Can you work these out from the model? Positions are in its coordinate system, mm. A direction names the side the tool comes from. Give positions to 0.01 mm unless a question says otherwise; leave off trailing zeros. Loops run counter-clockwise (first coordinate to the right, second up) from the corner with the lowest first, then second, coordinate; pieces in that order, holes last. Notation, with made-up numbers: M 7.25,-32.75 L 32.25,-32.75 A23 ccw 32.25,-7.75 Z; hole C 5,51 d6. An arc over 180 degrees is marked long. Put each result on its own line as item: value. Start each with the question number.
1) Imagine slicing it at B-B (z = 899). Write out the boundary of the cut face in (x, y), then the cut area to 3 significant figures.
2) For faces 5 (the cylindrical face through (378.69, -92.32, 749.78)), 6 (the flat face through (-317, -41, 865)), 7 (the flat face through (1, -39, 965)), 8 (the flat face through (-1, -55, 426)), 9 (the flat face through (313, -41, 865)), which set-ups out of +Z, -Z, +X, -X, +Y, -Y let a thin tool reach every point of the face, with its end or its side?
3) Imagine slicing it at A-A (y = -152.5). Write out the boundary of the cut face in (x, z).
4) For P1, Ø23.5, axis at x = -300, z = 662.5, coming from the -Y side; P2, Ø1, axis at x = -307.5, z = 209, coming from the -Y side; P3, Ø3, axis at x = 303.5, y = -105.5, coming from the +Z side, each with a flat end and sliding along its axis, tell me the tip position at first contact or that it passes through.
5) Imagine slicing it at C-C (z = 471.5). Write out the boundary of the cut face in (x, y), then the cut area to 3 significant figures.
6) If we mould it in two halves opening along X, with no side actions, what happens to faces 1 (the flat face through (310.4, -110, 147.9)), 2 (the cylindrical face through (-12.042, -92.325, 941.713)), 3 (the flat face through (-465, -39, 456)), 4 (the cylindrical face through (293.491, -107.465, 774.575))? For each: +X half, -X half, draft (parallel to the pull), parting line (faces both ways), or undercut.
7) Please list where these lines run through material, in increasing order: line 1 along Z through (x, y) = (0, -92.75); line 2 along X through (y, z) = (-84, 662); line 3 along Z through (x, y) = (-300, -50.5). Write a range as from..to.
8) Imagine slicing it at D-D (z = 276). Write out the boundary of the cut face in (x, y).
from build123d import *

# Parameters (mm, degrees)
F0_W      = 690
F0_H      = 350
F0_H_2    = 200
F1_DEPTH  = 80
F2_R      = 25
F2_R_2    = 75
F3_DEPTH  = 100
F4_R      = 75
F5_DEPTH  = 150
F6_R      = 82.5
F6_R_2    = 9
F6_R_3    = 25
F7_DEPTH  = 25
F8_R      = 50
F8_R_2    = 25
F9_DEPTH  = 5
F10_R     = 75
F11_DEPTH = 25
F12_R     = 37.5
F13_DEPTH = 100
F14_R     = 92.5
F14_R_2   = 9
F14_R_3   = 37.5
F15_DEPTH = 25
F16_R     = 60
F16_R_2   = 37.5
F17_DEPTH = 5
F18_W     = 930
F18_H     = 1000
F19_DEPTH = 100
F20_R     = 7
F21_DEPTH = 50
F22_W     = 300
F22_H     = 100
F23_DEPTH = 80


with BuildPart() as f1:
    # F0 (on Front) → F1 (new body)
    with BuildSketch(Plane.XZ):
        Polygon((345, -965), (465, -965), (465, 965), (-465, 965), (-465, -965), (-345, -965), (-345, -765), (345, -765), align=None)
        with Locations((0, -470)):
            Rectangle(F0_W, F0_H, mode=Mode.SUBTRACT)
        with Locations((0, -75)):
            Rectangle(F0_W, F0_H_2, mode=Mode.SUBTRACT)
    extrude(amount=F1_DEPTH)

    # F2 (on face) → F3 (cut)
    with BuildSketch(Plane.XZ.offset(80)):
        with Locations((-300, 125)):
            Circle(F2_R)
        with Locations((0, 425)):
            Circle(F2_R_2)
        with Locations((-300, 725)):
            Circle(F2_R)
        with Locations((300, 125)):
            Circle(F2_R)
        with Locations((300, 725)):
            Circle(F2_R)
    extrude(amount=-F3_DEPTH, mode=Mode.SUBTRACT)

    # F4 (on face) → F5 (join)
    with BuildSketch(Plane.XZ.offset(80)):
        with Locations((-370, 415)):
            Circle(F4_R)
        with Locations((370, 415)):
            Circle(F4_R)
    extrude(amount=F5_DEPTH)

    # F6 (on face) → F7 (join)
    with BuildSketch(Plane.XZ.offset(80)):
        with Locations((-300, 725)):
            Circle(F6_R)
        with Locations((-300, 662.5)):
            Circle(F6_R_2, mode=Mode.SUBTRACT)
        with Locations((-362.5, 725)):
            Circle(F6_R_2, mode=Mode.SUBTRACT)
        with Locations((-300, 725)):
            Circle(F6_R_3, mode=Mode.SUBTRACT)
        with Locations((-300, 787.5)):
            Circle(F6_R_2, mode=Mode.SUBTRACT)
        with Locations((-237.5, 725)):
            Circle(F6_R_2, mode=Mode.SUBTRACT)
        with Locations((-300, 125)):
            Circle(F6_R)
        with Locations((-300, 62.5)):
            Circle(F6_R_2, mode=Mode.SUBTRACT)
        with Locations((-362.5, 125)):
            Circle(F6_R_2, mode=Mode.SUBTRACT)
        with Locations((-300, 125)):
            Circle(F6_R_3, mode=Mode.SUBTRACT)
        with Locations((-237.5, 125)):
            Circle(F6_R_2, mode=Mode.SUBTRACT)
        with Locations((-300, 187.5)):
            Circle(F6_R_2, mode=Mode.SUBTRACT)
        with Locations((300, 725)):
            Circle(F6_R)
        with Locations((300, 662.5)):
            Circle(F6_R_2, mode=Mode.SUBTRACT)
        with Locations((237.5, 725)):
            Circle(F6_R_2, mode=Mode.SUBTRACT)
        with Locations((300, 725)):
            Circle(F6_R_3, mode=Mode.SUBTRACT)
        with Locations((362.5, 725)):
            Circle(F6_R_2, mode=Mode.SUBTRACT)
        with Locations((300, 787.5)):
            Circle(F6_R_2, mode=Mode.SUBTRACT)
        with Locations((300, 125)):
            Circle(F6_R)
        with Locations((237.5, 125)):
            Circle(F6_R_2, mode=Mode.SUBTRACT)
        with Locations((300, 62.5)):
            Circle(F6_R_2, mode=Mode.SUBTRACT)
        with Locations((300, 125)):
            Circle(F6_R_3, mode=Mode.SUBTRACT)
        with Locations((362.5, 125)):
            Circle(F6_R_2, mode=Mode.SUBTRACT)
        with Locations((300, 187.5)):
            Circle(F6_R_2, mode=Mode.SUBTRACT)
    extrude(amount=F7_DEPTH)

    # F8 (on face) → F9 (join)
    with BuildSketch(Plane.XZ.offset(105)):
        with Locations((-300, 725)):
            Circle(F8_R)
        with Locations((-300, 725)):
            Circle(F8_R_2, mode=Mode.SUBTRACT)
        with Locations((-300, 125)):
            Circle(F8_R)
        with Locations((-300, 125)):
            Circle(F8_R_2, mode=Mode.SUBTRACT)
        with Locations((300, 725)):
            Circle(F8_R)
        with Locations((300, 725)):
            Circle(F8_R_2, mode=Mode.SUBTRACT)
        with Locations((300, 125)):
            Circle(F8_R)
        with Locations((300, 125)):
            Circle(F8_R_2, mode=Mode.SUBTRACT)
    extrude(amount=F9_DEPTH)

    # F10 (on face) → F11 (join)
    with BuildSketch(Plane.XZ.offset(80)):
        with Locations((0, 425)):
            Circle(F10_R)
    extrude(amount=-F11_DEPTH)

    # F12 (on face) → F13 (cut)
    with BuildSketch(Plane.XZ.offset(80)):
        with Locations((0, 850)):
            Circle(F12_R)
    extrude(amount=-F13_DEPTH, mode=Mode.SUBTRACT)

    # F14 (on face) → F15 (join)
    with BuildSketch(Plane.XZ.offset(80)):
        with Locations((0, 850)):
            Circle(F14_R)
        with Locations((-72.5, 850)):
            Circle(F14_R_2, mode=Mode.SUBTRACT)
        with Locations((0, 777.5)):
            Circle(F14_R_2, mode=Mode.SUBTRACT)
        with Locations((0, 850)):
            Circle(F14_R_3, mode=Mode.SUBTRACT)
        with Locations((0, 922.5)):
            Circle(F14_R_2, mode=Mode.SUBTRACT)
        with Locations((72.5, 850)):
            Circle(F14_R_2, mode=Mode.SUBTRACT)
    extrude(amount=F15_DEPTH)

    # F16 (on face) → F17 (join)
    with BuildSketch(Plane.XZ.offset(105)):
        with Locations((0, 850)):
            Circle(F16_R)
        with Locations((0, 850)):
            Circle(F16_R_2, mode=Mode.SUBTRACT)
    extrude(amount=F17_DEPTH)

    # F18 (on face) → F19 (cut)
    with BuildSketch(Plane.XZ.offset(80)):
        with Locations((0, -465)):
            Rectangle(F18_W, F18_H)
    extrude(amount=-F19_DEPTH, mode=Mode.SUBTRACT)

    # F20 (on face) → F21 (cut)
    with BuildSketch(Plane(origin=(0, 0, 35), x_dir=(1, 0, 0), z_dir=(0, 0, -1))):
        with Locations((-400, 40)):
            Circle(F20_R)
        with Locations((400, 40)):
            Circle(F20_R)
    extrude(amount=-F21_DEPTH, mode=Mode.SUBTRACT)

    # F22 (on face) → F23 (cut)
    with BuildSketch(Plane.XZ.offset(80)):
        with Locations((-315, 915)):
            Rectangle(F22_W, F22_H)
        Polygon((-98.6675041929, 965), (-165, 965), (-165, 865), align=None)
        with Locations((315, 915)):
            Rectangle(F22_W, F22_H)
        Polygon((165, 865), (165, 965), (98.6675041929, 965), align=None)
    extrude(amount=-F23_DEPTH, mode=Mode.SUBTRACT)


solid = f1.part
Recorded:
1. outline: M -142.45,-80 L -78.46,-80 L -78.46,-105 L -34.63,-105 L -34.63,-110 L 34.63,-110 L 34.63,-105 L 78.46,-105 L 78.46,-80 L 142.45,-80 L 142.45,0 L -142.45,0 Z
1. area: 27,100 mm²
2. face 5: -Y
2. face 6: +Z, -X, +Y, -Y
2. face 7: +Z, +X, -X, +Y, -Y
2. face 8: +Y
2. face 9: +Z, +X, +Y, -Y
3. outline: C -370,415 d150; C 370,415 d150
4. P1: y = -105
4. P2: y = -80
4. P3: z = 807.47
5. outline: M -465,-80 L -419.32,-80 L -419.32,-230 L -320.68,-230 L -320.68,-80 L 320.68,-80 L 320.68,-230 L 419.32,-230 L 419.32,-80 L 465,-80 L 465,0 L 58.85,0 L 58.85,-55 L -58.85,-55 L -58.85,0 L -465,0 Z
5. area: 97,500 mm²
6. face 1: draft
6. face 2: undercut
6. face 3: -X half
6. face 4: undercut
7. line 1: 757.5..768.5, 786.5..812.5, 887.5..913.5, 931.5..942.5
7. line 2: -353.27..-308.99, -291.01..-246.73, 246.73..291.01, 308.99..353.27
7. line 3: 35..100, 150..700, 750..865
8. outline: M -465,-80 L 465,-80 L 465,0 L -465,0 Z
